The figure shows three views and two pictorial views of one solid part (mm, origin at its lowest corner). Answer the questions. A direction names the side the tool comes from. Round coordinates to 2 decimals unless told otherwise and drop trailing zeros. Order: outer loops, then holes, each group sorted by start corner. A loop starts at its lowest first (then second) coordinate and runs counter-clockwise, first axis right, second up. Notation, with made-up numbers: (-33.75, 28) - (-29.75, 28) arc R31 cw to (-29.75, 62) - close; hole circle Ø4 at (43, -22.5). An arc over 180 degrees is marked (long way). Answer in a Markdown table with one row per item.
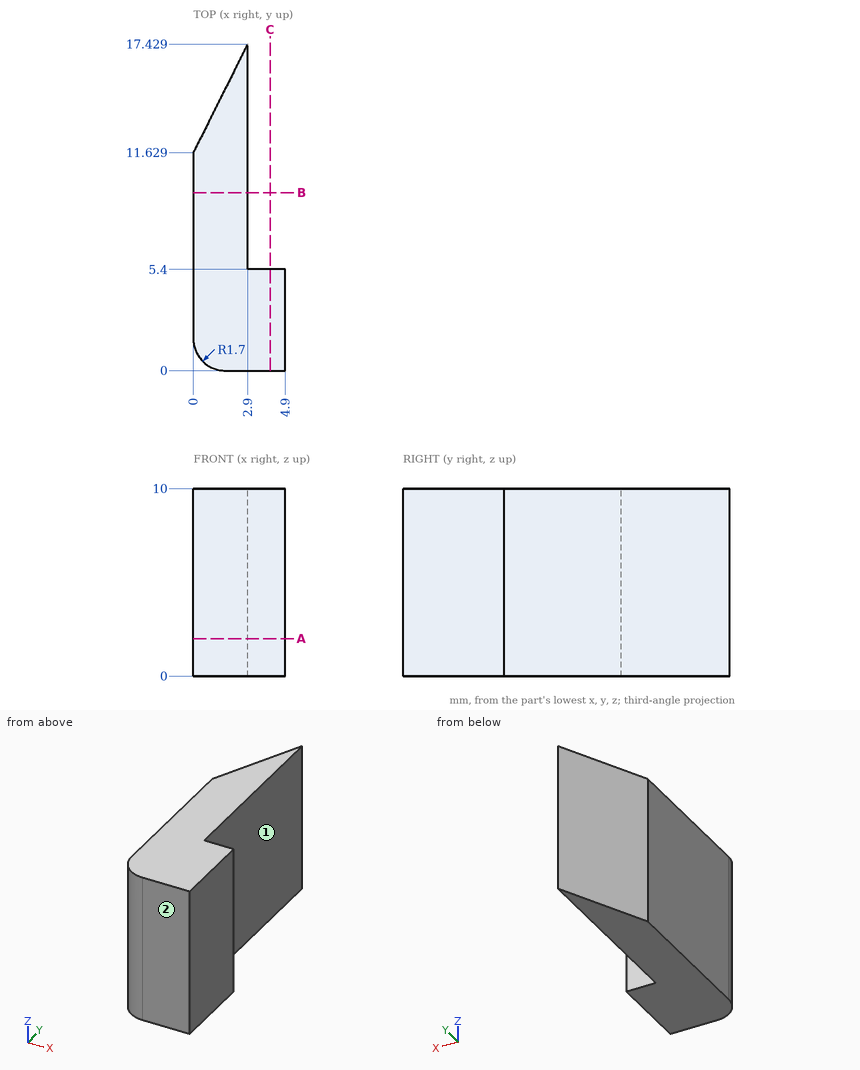
1) Find section A-A, the plane z = 2. Give the vertices of the cut face in (x, y), then the cut area to 3 significant figures.
Filled in:
| item | result |
|---|---|
| outline | (0, 1.7) arc R1.7 ccw to (1.7, 0) - (4.9, 0) - (4.9, 5.4) - (2.9, 5.4) - (2.9, 17.43) - (0, 11.63) - close |
| area | 52.3 mm^2 |
2) Find section C-C, the plane x = 4.1. Give the vertices of the cut face in (y, z), then the cut area to 3 significant figures.
Filled in:
| item | result |
|---|---|
| outline | (0, 0) - (5.4, 0) - (5.4, 10) - (0, 10) - close |
| area | 54.0 mm^2 |
3) Find the intervals of material crossed by probe 1 along X at (y, z) = (11.25, 6); probe 2 along Y at (x, z) = (4.15, 6.25); probe 3 along Y at (x, z) = (1.55, 6.25) (1 decimal), in increasing order. Write a range as from..to.
Filled in:
| item | result |
|---|---|
| probe 1 | x = 0..2.9 |
| probe 2 | y = 0..5.4 |
| probe 3 | y = 0..14.7 |
4) Which of the six approach directions +Z, -Z, +X, -X, +Y, -Y give full straight-line access (tool end or side, diameter ignored) to the marked faces 1 and 2?
Filled in:
| item | result |
|---|---|
| face 1 | +Z, -Z, +X, +Y |
| face 2 | +Z, -Z, +X, -X, -Y |
5) Find section B-B, the plane y = 9.5. Give the vertices of the cut face in (x, z).
Filled in:
| item | result |
|---|---|
| outline | (0, 0) - (2.9, 0) - (2.9, 10) - (0, 10) - close |
6) Each of these flat-tipped pins is pushed along its axis until it touches: pin 1 (1 mm diameter, centred on y = 11.5, z = 4, fed in from +X); pin 2 (2 mm diameter, centred on x = 4, z = 7, fed in from +Y); pin 3 (1 mm diameter, centred on y = 12.5, z = 3, fed in from -X) (1 decimal). Where does it stop, or does it pass through?
Filled in:
| item | result |
|---|---|
| pin 1 | stops at x = 2.9 |
| pin 2 | stops at y = 5.4 |
| pin 3 | stops at x = 0.2 |
